Model file for the job. Use its own axes, mm. A direction names the side the tool comes from. Coordinates: 2 decimals unless noted, no trailing zeros.
from build123d import *

# Parameters (mm, degrees)
SKETCH3_R           = 9.271
BOSS_EXTRUDE1_DEPTH = 3.175
FILLET1_R           = 0.254


with BuildPart() as part:
    # Sketch2 → Revolve5 (revolve)
    with BuildSketch(Plane(origin=(0, 0, 0.100515376), x_dir=(1, 0, 0), z_dir=(0, 1, 0))):
        with BuildLine():
            Line((0, 0), (0, 25.4))
            Line((0, 25.4), (12.7, 25.4))
            add(Edge.make_bspline(
                [(0, 0), (4.251787512, -0.000213004), (11.607750415, 10.081742809), (12.7, 23.292671224), (12.7, 25.4)],
                knots=[0.5, 0.5, 0.5, 0.5, 0.789002784, 1, 1, 1, 1], degree=3))
        make_face()
    revolve(axis=Axis((0, 0, 0.100515376), (0, 0, -1)))

    # Sketch3 → Boss-Extrude1 (add)
    with BuildSketch(Plane(origin=(0, 0, -25.299484624), x_dir=(-1, 0, 0), z_dir=(0, 0, -1))):
        Circle(SKETCH3_R)
    extrude(amount=BOSS_EXTRUDE1_DEPTH)

    # Fillet1
    fillet1_edges = [part.edges().sort_by_distance(p)[0] for p in [
        (9.271, 0, -25.299484624),
    ]]
    fillet(fillet1_edges, radius=FILLET1_R)

    # Chamfer1: read off the stored shape, not the designer's step
    # Chamfer1 outline → Chamfer1 (revolve, cut)
    with BuildSketch(Plane.XZ):
        Polygon((9.271, -28.220484624), (9.017, -28.474484624), (9.271, -28.474484624), align=None)
        Polygon((12.698013115, -25.047471509), (12.446, -25.299484624), (12.698013115, -25.299484624), align=None)
    revolve(axis=Axis((0, 0, 0), (0, 0, 1)), mode=Mode.SUBTRACT)

    # Chamfer1 2 outline → Chamfer1 2 (revolve, cut)
    with BuildSketch(Plane.XZ):
        with BuildLine():
            add(Edge.make_bspline(
                [(12.698013115, -25.047471509), (12.699349278, -25.136229047), (12.7, -25.220304585), (12.7, -25.299484624)],
                knots=[0.992072064, 0.992072064, 0.992072064, 0.992072064, 1, 1, 1, 1], degree=3))
            Line((12.698013115, -25.047471509), (12.698013115, -25.299484624))
            Line((12.698013115, -25.299484624), (12.7, -25.299484624))
        make_face()
    revolve(axis=Axis((0, 0, 0), (0, 0, 1)), mode=Mode.SUBTRACT)


solid = part.part
Q1. Drill centre lines: line 1 (Z direction, x = -3.75, y = 8.75); line 2 (X direction, y = -6.5, z = -10); line 3 (X direction, y = 0.25, z = -4.5). Where is each one in solid material? Low to high.
Answers:
line 1: z = -25.3 to -9.51
line 2: x = -7.24 to 7.24
line 3: x = -6.74 to 6.74
Q2. Which spindle directions (+Z, -Z, +X, -X, +Y, -Y) get a long thin tool onto all of the face, cutting with end or side? Do faces 1 (the flat face through (0, 0, -28.474)), 2 (the cylindrical face through (6.8, 6.3, -26.9)). Say none if no direction does.
Answers:
face 1: -Z, +X, -X, +Y, -Y
face 2: -Z
Q3. Flat gauge pins, fed straight in: P1, Ø3, axis at x = 6.5, z = -11.5, coming from the +Y side; P2, Ø10, axis at x = -4.5, y = 6, coming from the +Z side; P3, Ø5, axis at x = 8, z = -11.5, coming from the +Y side. Where does each tip first touch, or does it go through?
Answers:
P1: stops at y = 9.18
P2: stops at z = -0.54
P3: stops at y = 8.98
